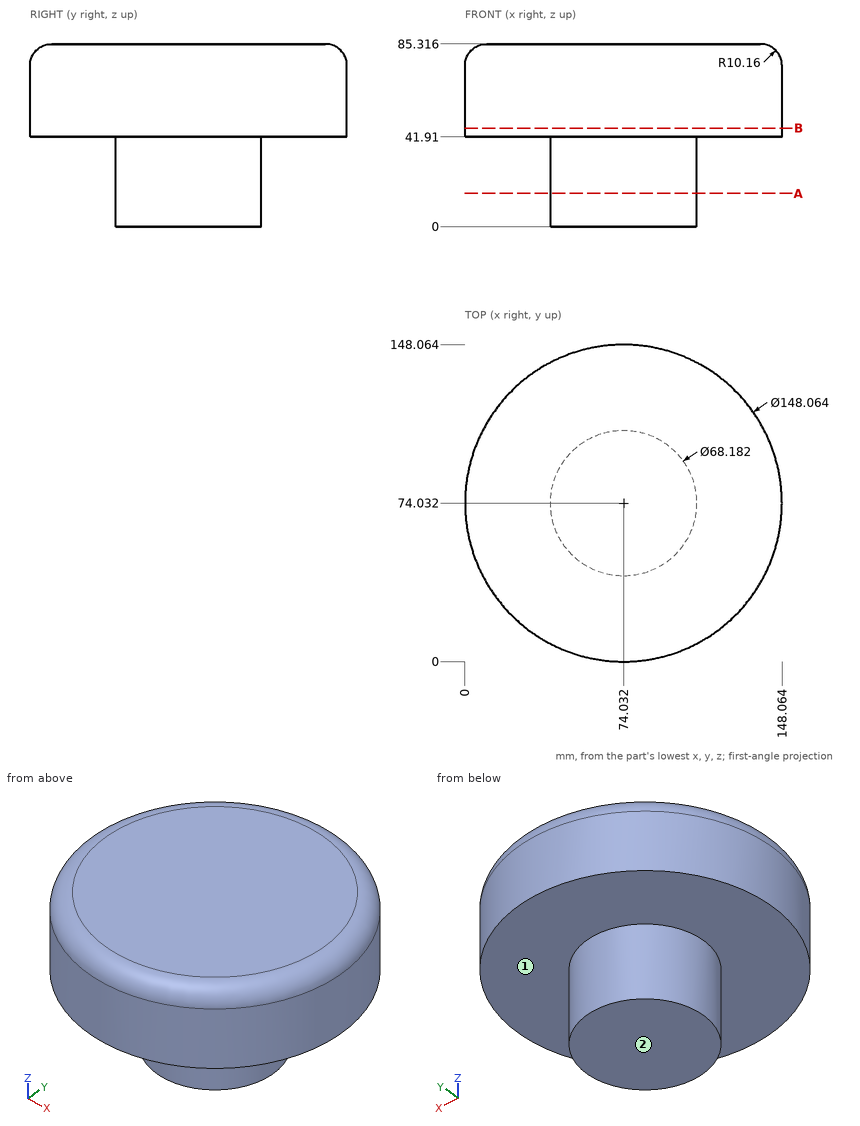
Study the drawing (mm; zero at the part's minimum x, y, z) and answer. A direction names the side the tool comes from. Coordinates: 2 decimals unless noted, no trailing zeros. Loops run counter-clockwise (first coordinate to the right, second up) from the corner with the lowest first, then second, coordinate; pieces in that order, holes last. Notation, with made-up numbers: (31, 3.5) -> (85, 3.5) arc R17 ccw to (85, 9.5) -> close; hole circle Ø6 at (-38, 14.5). An arc over 180 degrees is marked (long way). Write item = value, one per line. Start each with the question number.
1) The part is cut by section B-B, the plane z = 46. Determine the outline of the cut face in (x, y), plus the area to 3 significant figures.
2) The part is cut by section A-A, the plane z = 15.5. Determine the outline of the cut face in (x, y), plus the area to 3 significant figures.
3) Given P1, Ø6, axis at x = 57.5, z = 20, coming from the +Y side; P2, Ø8, axis at y = 39, z = 44, coming from the -X side; P3, Ø12, axis at x = 71.5, z = 62.5, coming from the +Y side, each flat-ended and moving along its own axis, determine where each tip first touches the part or whether it passes through.
4) Find the intervals of material crossed by L1, parallel to Z at x = 54, y = 111.5 (1 decimal); L2, parallel to Y at x = 74, z = 52; L3, parallel to Y at x = 91.5, z = 54.5, in increasing order. Write a range as from..to.
5) For the marked faces 1 and 2, determine the directions among +Z, -Z, +X, -X, +Y, -Y from which every point of the face is accessible in a straight line to the end or side of a thin tool.
Result:
q1.outline = circle Ø148.06 at (74.03, 74.03)
q1.area = 17,200 mm²
q2.outline = circle Ø68.18 at (74.03, 74.03)
q2.area = 3,650 mm²
q3.P1 = 105.32
q3.P2 = 6.82
q3.P3 = 148.06
q4.L1 = 41.9..85.3
q4.L2 = 0..148.06
q4.L3 = 2.09..145.97
q5.face_1 = -Z
q5.face_2 = -Z, +X, -X, +Y, -Y
